Verification items for the finished model (mm, model axes). A direction names the side the tool comes from. Coordinates: 2 decimals unless noted, no trailing zeros. Loops run counter-clockwise (first coordinate to the right, second up) from the corner with the lowest first, then second, coordinate; pieces in that order, holes last. Notation, with made-up numbers: (-8.75, 63.5) -> (42.25, 63.5) arc R16 ccw to (42.25, 85.5) -> close; hole circle Ø2 at (40, 41). An arc over 180 degrees is marked (long way). Answer as a JSON object with one key per item and string values. Group by question number.
Q1. Cross-section at A-A on y = -401.5. Record the boundary of the cut face in (x, z), and give its area (3 significant figures).
Q2. Gauge pin test, flat ends, axial feed: pin 1 Ø8.5 at (y, z) = (-245.5, 18) entering from -X; pin 2 Ø1 at (x, y) = (-7.5, -118.5) entering from -Z. Record the tip position at first contact, or that the pin passes through.
Q3. Set-up check for faces 1 (the flat face through (-11, -296, 28)), 2 (the flat face through (0, -296, 15)): record each of +Z, -Z, +X, -X, +Y, -Y from which the full face is reachable in a straight line by a thin tool's end or side.
Q4. Scan lines: L1, parallel to Y at x = -0.8, z = 10; L2, parallel to Z at x = -1, y = -10; L3, parallel to Z at x = -1.2, y = -30. Record each from-to range of solid material in increasing order.
Q5. Cross-section at B-B on x = -5.5. Record the boundary of the cut face in (y, z), and give its area (3 significant figures).
```python
from build123d import *

# Parameters (mm, degrees)
PAD_DEPTH   = 600
SKETCH001_R = 3.25
HOLE_DEPTH  = 25


with BuildPart() as part:
    # Sketch → Pad (new body)
    with BuildSketch(Plane.XZ):
        Polygon((-20, 30), (0, 30), (0, 0), (-2, 0), (-2, 28), (-20, 28), align=None)
    extrude(amount=PAD_DEPTH)

    # Sketch001 (on Face4 of Pad) → Hole (cut)
    with BuildSketch(Plane(origin=(-2, 0, 0), x_dir=(0, 0, -1), z_dir=(-1, 0, 0))):
        with Locations((-18, 10)):
            Circle(SKETCH001_R)
        with Locations((-10, 30)):
            Circle(SKETCH001_R)
        with Locations((-10, 590)):
            Circle(SKETCH001_R)
        with Locations((-20, 570)):
            Circle(SKETCH001_R)
    extrude(amount=-HOLE_DEPTH, mode=Mode.SUBTRACT)


solid = part.part
```
Computed values:
{
 "1": {"outline": "(-20, 28) -> (-2, 28) -> (-2, 0) -> (0, 0) -> (0, 30) -> (-20, 30) -> close", "area": "96.0 mm²"},
 "2": {"pin 1": "stops at x = -2", "pin 2": "stops at z = 28"},
 "3": {"face 1": "-Z, -X, +Y, -Y", "face 2": "+Z, -Z, +X, +Y, -Y"},
 "4": {"L1": "y = -600 to -593.25, -586.75 to -33.25, -26.75 to 0", "L2": "z = 0 to 14.75, 21.25 to 30", "L3": "z = 0 to 6.75, 13.25 to 30"},
 "5": {"outline": "(-600, 28) -> (0, 28) -> (0, 30) -> (-600, 30) -> close", "area": "1,200 mm²"}
}
